For this review, take the finished solid that the model builds, in its own axes (mm). Face numbers are marked on the shaded views. Give positions to 0.01 mm unless a question says otherwise; leave off trailing zeros. Order: outer loops, then holes, each group sorted by start corner. A loop starts at its lowest first (then second) coordinate and runs counter-clockwise, first axis right, second up. Notation, with made-up numbers: (27.25, -27) -> (35.25, -27) arc R17 ccw to (35.25, -10) -> close; hole circle Ø11 at (-12, -27.5). An arc over 180 degrees is marked (long way). One line per item, written item: value. Start each with the question number.
Autodesk Inventor part; units mm, degrees
ref_plane "YZ Plane" through (0, 0, 0) normal (1, 0, 0) x (0, 1, 0)
ref_plane "XZ Plane" through (0, 0, 0) normal (0, 1, 0) x (-1, 0, 0)
ref_plane "XY Plane" through (0, 0, 0) normal (0, 0, 1) x (1, 0, 0)
sketch "スケッチ1" plane through (0, 0, 0) normal (0, 0, 1) x (1, 0, 0)
  line L0 (-28, -39.55) -> (28, -39.55) construction
  line L1 (28, -39.55) -> (28, 39.55) construction
  line L2 (28, 39.55) -> (-28, 39.55) construction
  line L3 (-28, 39.55) -> (-28, -39.55) construction
  line L4 (-28, -39.55) -> (28, 39.55) construction
  line L5 (28, -39.55) -> (-28, 39.55) construction
  line L6 (-28, 26.65) -> (-28, 39.55)
  line L7 (-28, 39.55) -> (28, 39.55)
  line L8 (28, 39.55) -> (28, 26.65)
  line L9 (-28, 24.55) -> (-33, 24.55)
  line L10 (-33, 24.55) -> (-33, -24.55)
  line L11 (-33, -24.55) -> (-28, -24.55)
  line L12 (-28, -26.65) -> (-28, -39.55)
  line L13 (-28, -39.55) -> (28, -39.55)
  line L14 (28, -39.55) -> (28, -26.65)
  line L15 (28, 24.55) -> (33, 24.55)
  line L16 (33, 24.55) -> (33, -24.55)
  line L17 (33, -24.55) -> (28, -24.55)
  arc A0 (-28, 24.55) -> (-28, 26.65) centre (-28, 25.6) ccw
  arc A1 (-28, -26.65) -> (-28, -24.55) centre (-28, -25.6) ccw
  arc A2 (28, -24.55) -> (28, -26.65) centre (28, -25.6) ccw
  line L18 (0, 0) -> (0, 39.55) construction
  line L19 (0, 0) -> (28, 0) construction
  arc A3 (28, 26.65) -> (28, 24.55) centre (28, 25.6) ccw
  dimension "d9" = 56
  dimension "d12" = 79.1
  dimension "d13" = 15
  dimension "d39" = 15
  dimension "d40" = 1.05
  dimension "d41" = 5
extrude "押し出し1" add sketch "スケッチ1" along normal blind 5
sketch "スケッチ2" plane through (0, 0, 5) normal (0, 0, 1) x (1, 0, 0)
  line L0 (-28, 39.55) -> (-28, 26.65)
  line L1 (28, 39.55) -> (-28, 39.55)
  line L2 (-67.7785, 43.014) -> (-28, 43.014)
  line L3 (-28, 43.014) -> (-28, -43.014)
  line L4 (-28, -43.014) -> (-67.7785, -43.014)
  line L5 (-67.7785, -43.014) -> (-67.7785, 43.014)
  line L6 (67.7785, 43.014) -> (28, 43.014)
  line L7 (28, 43.014) -> (28, -43.014)
  line L8 (28, -43.014) -> (67.7785, -43.014)
  line L9 (67.7785, -43.014) -> (67.7785, 43.014)
  line L10 (0, 0) -> (0, 39.55) construction
  line L11 (0, 0) -> (33, 0) construction
  line L12 (33, 24.55) -> (33, -24.55) construction
extrude "押し出し2" cut sketch "スケッチ2" against normal blind 2.5
sketch "スケッチ3" plane through (0, 0, 5) normal (0, 0, 1) x (1, 0, 0)
  line L0 (28, 39.55) -> (-28, 39.55)
  line L1 (-28, 39.55) -> (-28, 26.65)
  line L2 (-20, -31.55) -> (20, -31.55)
  line L3 (20, -31.55) -> (20, 31.55)
  line L4 (20, 31.55) -> (-20, 31.55)
  line L5 (-20, 31.55) -> (-20, -31.55)
  line L6 (-20, -31.55) -> (20, 31.55) construction
  line L7 (20, -31.55) -> (-20, 31.55) construction
  point P0 (0, 0)
  dimension "d47" = 8
  dimension "d48" = 8
extrude "押し出し3" cut sketch "スケッチ3" against normal blind 10
fillet "フィレット1" radius 10 4 edges at (-20, 31.55, 2.5) (20, 31.55, 2.5) (20, -31.55, 2.5) (-20, -31.55, 2.5)
equation "\"d12\" = d18"
equation "\"d13\" = d28"
equation "\"d39\" = d13"
equation "\"d47\" = d48"
properties part number "コックピット_2_サブフレーム_1" material "アセタール樹脂、黒"
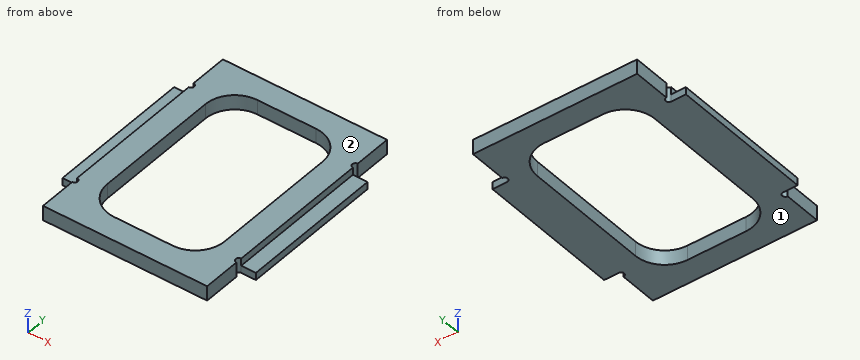
Q1. Mouldability with a two-part tool opening along Z and no side actions: class the marked faces 1 and 2 as pulls with the +Z half, pulls with the -Z half, needs draft (parallel to the pull), parting line crosses it, or undercut.
Q2. Take a section at A-A (y = 9.5). State the section outline as (x, z) points, and give its area (3 significant figures).
Q3. Take a section at B-B (z = 4.1). State the section outline as (x, y) points.
Q4. Take a section at D-D (y = 25.6). State the section outline as (x, z) points, and give its area (3 significant figures).
Q5. For line 1 along Y through (x, z) = (-3.5, 3.95); line 2 along X through (y, z) = (19.5, 4.1); line 3 along X through (y, z) = (-4, 0.3), list the stretches that pass through material, from the lowest coordinate up.
Q6. For pin 1 Ø2.5 at (x, y) = (31, -10.5) entering from +Z; pin 2 Ø3 at (x, z) = (30, 1.5) entering from -Y; pin 3 Ø0.8 at (x, z) = (30.5, 1) entering from +Y, all flat-tipped, find the tip position at first contact; note any pin that passes through.
Q7. Take a section at C-C (x = 16). State the section outline as (y, z) points, and give its area (4 significant figures).
Answers below:
1. face 1: pulls with the -Z half
1. face 2: pulls with the +Z half
2. outline: (-33, 0) -> (-20, 0) -> (-20, 5) -> (-28, 5) -> (-28, 2.5) -> (-33, 2.5) -> close; (20, 0) -> (33, 0) -> (33, 2.5) -> (28, 2.5) -> (28, 5) -> (20, 5) -> close
2. area: 105 mm²
3. outline: (-28, -39.55) -> (28, -39.55) -> (28, -26.65) arc R1.05 cw to (28, -24.55) -> (28, 24.55) arc R1.05 cw to (28, 26.65) -> (28, 39.55) -> (-28, 39.55) -> (-28, 26.65) arc R1.05 cw to (-28, 24.55) -> (-28, -24.55) arc R1.05 cw to (-28, -26.65) -> close; hole (-20, -21.55) arc R10 ccw to (-10, -31.55) -> (10, -31.55) arc R10 ccw to (20, -21.55) -> (20, 21.55) arc R10 ccw to (10, 31.55) -> (-10, 31.55) arc R10 ccw to (-20, 21.55) -> close
4. outline: (-26.95, 0) -> (-19.14, 0) -> (-19.14, 5) -> (-26.95, 5) -> close; (19.14, 0) -> (26.95, 0) -> (26.95, 5) -> (19.14, 5) -> close
4. area: 78.1 mm²
5. line 1: y = -39.55 to -31.55, 31.55 to 39.55
5. line 2: x = -28 to -20, 20 to 28
5. line 3: x = -33 to -20, 20 to 33
6. pin 1: stops at z = 2.5
6. pin 2: stops at y = -24.55
6. pin 3: stops at y = 24.55
7. outline: (-39.55, 0) -> (-29.55, 0) -> (-29.55, 5) -> (-39.55, 5) -> close; (29.55, 0) -> (39.55, 0) -> (39.55, 5) -> (29.55, 5) -> close
7. area: 100.0 mm²
